Job drawing, mm, ordinate dimensions from the low corner. One solid piece. A direction names the side the tool comes from. Round coordinates to 2 decimals unless told otherwise and drop trailing zeros. Write each loop counter-clockwise with the first axis right and the second up, starting at its lowest first coordinate (ties: lowest second). Pieces come first, ordered by that corner, then holes. Notation, with made-up numbers: M 68.5,-38.75 L 116.5,-38.75 A9 cw 116.5,-31.75 Z; hole C 60,-27 d2. An arc over 180 degrees is marked long. Answer as a JSON object with one key per item and string values. Group by question number.
1. Band-saw the part on B-B, the plane y = 11.3. Write the cut outline in (x, z), plus the area to 3 significant figures.
2. Which spindle directions (+Z, -Z, +X, -X, +Y, -Y) get a long thin tool onto all of the face, cutting with end or side? Do the marked faces 1 and 2. Say none if no direction does.
3. Band-saw the part on D-D, the plane y = 16.5. Write the cut outline in (x, z).
4. Drop flat-ended pins along their axis: pin 1 (5 mm diameter, centred on x = 18.5, y = 10.5, fed in from -Z); pin 2 (2 mm diameter, centred on x = 2.5, y = 2.5, fed in from -Z). Give the stop position or say it passes through.
5. Band-saw the part on C-C, the plane z = 4. Write the cut outline in (x, y).
6. Band-saw the part on A-A, the plane x = 44. Write the cut outline in (y, z).
7. Drill centre lines: line 1 (Y direction, x = 16, z = 4.5); line 2 (X direction, y = 7.5, z = 9.25). Where is each one in solid material? Low to high. Write a range as from..to.
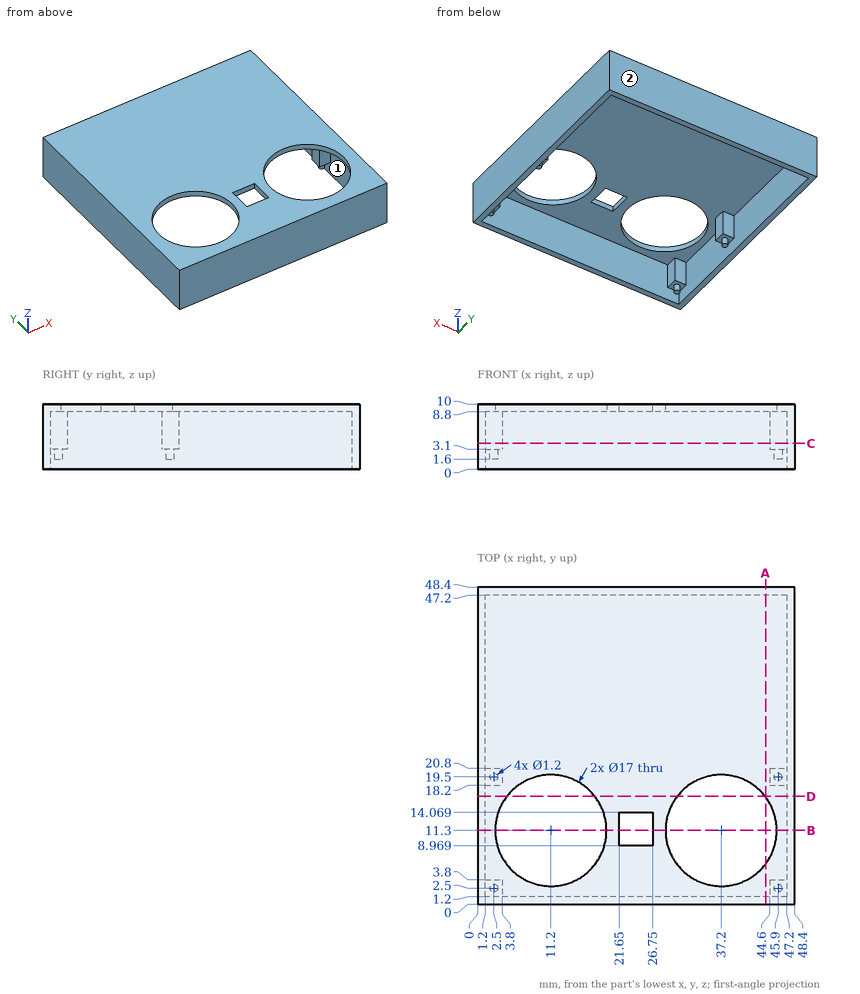
Worked answers:
{
 "1": {"outline": "M 0,0 L 1.2,0 L 1.2,8.8 L 2.7,8.8 L 2.7,10 L 0,10 Z; M 19.7,8.8 L 21.65,8.8 L 21.65,10 L 19.7,10 Z; M 26.75,8.8 L 28.7,8.8 L 28.7,10 L 26.75,10 Z; M 45.7,8.8 L 47.2,8.8 L 47.2,0 L 48.4,0 L 48.4,10 L 45.7,10 Z", "area": "32.3 mm^2"},
 "2": {"face 1": "-Z", "face 2": "+Z, -Z, +X, -X, +Y"},
 "3": {"outline": "M 0,0 L 1.2,0 L 1.2,8.8 L 4.48,8.8 L 4.48,10 L 0,10 Z; M 17.92,8.8 L 30.48,8.8 L 30.48,10 L 17.92,10 Z; M 43.92,8.8 L 47.2,8.8 L 47.2,0 L 48.4,0 L 48.4,10 L 43.92,10 Z"},
 "4": {"pin 1": "stops at z = 8.8", "pin 2": "stops at z = 1.6"},
 "5": {"outline": "M 0,0 L 48.4,0 L 48.4,48.4 L 0,48.4 Z; hole M 1.2,3.8 L 3.8,3.8 L 3.8,1.2 L 44.6,1.2 L 44.6,3.8 L 47.2,3.8 L 47.2,18.2 L 44.6,18.2 L 44.6,20.8 L 47.2,20.8 L 47.2,47.2 L 1.2,47.2 L 1.2,20.8 L 3.8,20.8 L 3.8,18.2 L 1.2,18.2 Z"},
 "6": {"outline": "M 0,0 L 1.2,0 L 1.2,8.8 L 6.2,8.8 L 6.2,10 L 0,10 Z; M 16.4,8.8 L 47.2,8.8 L 47.2,0 L 48.4,0 L 48.4,10 L 16.4,10 Z"},
 "7": {"line 1": "y = 0..1.2, 47.2..48.4", "line 2": "x = 0..3.6, 18.8..29.6, 44.8..48.4"}
}
